Autodesk Inventor part; units mm, degrees
ref_plane "YZ Plane" through (0, 0, 0) normal (1, 0, 0) x (0, 1, 0)
ref_plane "XZ Plane" through (0, 0, 0) normal (0, 1, 0) x (-1, 0, 0)
ref_plane "XY Plane" through (0, 0, 0) normal (0, 0, 1) x (1, 0, 0)
sketch "Sketch1" plane through (0, 0, 0) normal (0, 1, 0) x (-1, 0, 0)
  arc A0 (32.2948, 13.759) -> (-8.6569, 13.759) centre (11.8189, 4.9346) ccw
  line L0 (-8.6569, 13.759) -> (-8.6569, -3.8898)
  line L1 (-1.7811, -3.8898) -> (-8.6569, -3.8898)
  line L2 (-1.7811, -3.8898) -> (-1.7811, -10.2398)
  line L3 (-1.7811, -10.2398) -> (4.2189, -10.2398)
  line L4 (4.2189, -10.2398) -> (4.2189, -3.8898)
  line L5 (10.3189, -3.8898) -> (4.2189, -3.8898)
  line L6 (10.3189, -3.8898) -> (10.3189, 2.1102)
  line L7 (10.3189, 2.1102) -> (9.0689, 2.1102)
  line L8 (9.0689, 2.1102) -> (9.0689, 4.1102)
  line L9 (9.0689, 4.1102) -> (10.3189, 4.1102)
  line L10 (10.3189, 4.1102) -> (10.3189, 6.7602)
  line L11 (10.3189, 6.7602) -> (13.3189, 6.7602)
  line L12 (13.3189, 6.7602) -> (13.3189, 4.1102)
  line L13 (13.3189, 4.1102) -> (14.5689, 4.1102)
  line L14 (14.5689, 4.1102) -> (14.5689, 2.1102)
  line L15 (14.5689, 2.1102) -> (13.3189, 2.1102)
  line L16 (13.3189, 2.1102) -> (13.3189, -3.8898)
  line L17 (19.4189, -3.8898) -> (13.3189, -3.8898)
  line L18 (19.4189, -3.8898) -> (19.4189, -10.2398)
  line L19 (19.4189, -10.2398) -> (25.4189, -10.2398)
  line L20 (25.4189, -10.2398) -> (25.4189, -3.8898)
  line L21 (32.2948, -3.8898) -> (25.4189, -3.8898)
  line L22 (32.2948, -3.8898) -> (32.2948, 13.759)
  circle A1 centre (11.8189, 11.3099) radius 4
  line L23 (-7.9734, -40.7116) -> (-7.9734, -55.3652)
  line L24 (-1.0976, -55.3652) -> (-7.9734, -55.3652)
  line L25 (-1.0976, -55.3652) -> (-1.0976, -61.7152)
  line L26 (-1.0976, -61.7152) -> (4.9025, -61.7152)
  line L27 (4.9025, -61.7152) -> (4.9025, -55.3652)
  line L28 (11.0025, -55.3652) -> (4.9025, -55.3652)
  line L29 (11.0025, -55.3652) -> (11.0025, -49.3652)
  line L30 (11.0025, -49.3652) -> (9.7525, -49.3652)
  line L31 (9.7525, -49.3652) -> (9.7525, -47.3652)
  line L32 (9.7525, -47.3652) -> (11.0025, -47.3652)
  line L33 (11.0025, -47.3652) -> (11.0025, -44.7152)
  line L34 (11.0025, -44.7152) -> (14.0025, -44.7152)
  line L35 (14.0025, -44.7152) -> (14.0025, -47.3652)
  line L36 (14.0025, -47.3652) -> (15.2524, -47.3652)
  line L37 (15.2524, -47.3652) -> (15.2524, -49.3652)
  line L38 (15.2524, -49.3652) -> (14.0025, -49.3652)
  line L39 (14.0025, -49.3652) -> (14.0025, -55.3652)
  line L40 (20.1024, -55.3652) -> (14.0025, -55.3652)
  line L41 (20.1024, -55.3652) -> (20.1024, -61.7152)
  line L42 (20.1024, -61.7152) -> (26.1024, -61.7152)
  line L43 (26.1024, -61.7152) -> (26.1024, -55.3652)
  line L44 (32.9783, -55.3652) -> (26.1024, -55.3652)
  line L45 (32.9783, -55.3652) -> (32.9783, -40.7116)
  line L46 (32.9783, -40.7116) -> (-7.9734, -40.7116)
  point P0 (0, 0)
  point P1 (0.6835, -51.4754)
  point P2 (12.5025, -46.5408)
extrude "Extrusion1" add sketch "Sketch1" along normal blind 6 contours L46 L45 L44 L43 L42 L41 L40 L39 L38 L37 L36 L35 L34 L33 L32 L31 L30 L29 L28 L27 L26 L25 L24 L23
sketch "Sketch2" plane through (0, 6, 0) normal (0, 1, 0) x (1, 0, 0)
  line L0 (-14.0025, 49.3652) -> (-14.0025, 55.3652)
  line L1 (-15.2524, 47.3652) -> (-15.2524, 49.3652)
  line L2 (-15.2524, 49.3652) -> (-14.0025, 49.3652)
  line L3 (-14.0025, 47.3652) -> (-15.2524, 47.3652)
  line L4 (-14.0025, 44.7152) -> (-14.0025, 47.3652)
  line L5 (-11.0025, 44.7152) -> (-14.0025, 44.7152)
  line L6 (-11.0025, 47.3652) -> (-11.0025, 44.7152)
  line L7 (-9.7525, 47.3652) -> (-11.0025, 47.3652)
  line L8 (-9.7525, 49.3652) -> (-9.7525, 47.3652)
  line L9 (-11.0025, 49.3652) -> (-9.7525, 49.3652)
  line L10 (-11.0025, 55.3652) -> (-11.0025, 49.3652)
  line L11 (-4.9025, 55.3652) -> (-11.0025, 55.3652)
  line L12 (-11.0025, 55.3652) -> (-14.0025, 55.3652)
  line L13 (-14.2025, 47.1652) -> (-15.4524, 47.1652)
  line L14 (-15.4524, 47.1652) -> (-15.4524, 49.5652)
  line L15 (-15.4524, 49.5652) -> (-14.2025, 49.5652)
  line L16 (-14.2025, 49.5652) -> (-14.2025, 55.5652)
  line L17 (-14.2025, 55.5652) -> (-10.8025, 55.5652)
  line L18 (-10.8025, 55.5652) -> (-10.8025, 49.5652)
  line L19 (-10.8025, 49.5652) -> (-9.5525, 49.5652)
  line L20 (-9.5525, 49.5652) -> (-9.5525, 47.1652)
  line L21 (-9.5525, 47.1652) -> (-10.8025, 47.1652)
  line L22 (-10.8025, 47.1652) -> (-10.8025, 44.5152)
  line L23 (-10.8025, 44.5152) -> (-14.2025, 44.5152)
  line L24 (-14.2025, 44.5152) -> (-14.2025, 47.1652)
  point P0 (0, 0)
  dimension "d2" = 0.2
extrude "Extrusion2" cut sketch "Sketch2" against normal blind 25.4
sketch "Sketch3" plane through (0, 6, 0) normal (0, 1, 0) x (1, 0, 0)
  line L0 (2.9926, 65.1915) -> (-28.8734, 65.1915)
  line L1 (-28.8734, 65.1915) -> (-28.8734, 59.7152)
  line L2 (-28.8734, 59.7152) -> (2.9926, 59.7152)
  line L3 (2.9926, 59.7152) -> (2.9926, 65.1915)
  line L4 (-20.1024, 61.7152) -> (-26.1024, 61.7152)
  point P0 (0, 0)
  dimension "d5" = 2
extrude "Extrusion3" cut sketch "Sketch3" against normal blind 25.4
fillet "Fillet1" radius 0.5 4 edges at (-26.1024, 3, -59.7152) (-20.1024, 3, -59.7152) (-4.9025, 3, -59.7152) (1.0976, 3, -59.7152)
properties part number "Maker_jigsaw_template"
Can you work these out from the model? Positions are in its coordinate system, mm. A direction names the side the tool comes from. Round coordinates to 2 decimals unless told otherwise and drop trailing zeros. Loops run counter-clockwise (first coordinate to the right, second up) from the corner with the lowest first, then second, coordinate; pieces in that order, holes last. Notation, with made-up numbers: M 14,89.25 L 50,89.25 A29 cw 50,112.25 Z; hole C 23,-2 d11. An arc over 180 degrees is marked long. Answer as a JSON object with one key per item and string values. Group by question number.
Q1. Imagine slicing it at C-C, the plane z = -50. Please give me the cut outline in (x, y).
Q2. We'd pull the mould along X, two halves only. Please class faces 1 (the flat face through (-13, 3, -40.712)), 2 (the flat face through (-26.102, 3, -57)), 3 (the flat face through (1.098, 3, -57)), 4 (the flat face through (-10, 3, -49.565)): +X half, -X half, draft (parallel to the pull), parting line (faces both ways), or undercut.
Q3. On a 3-axis mill with a long thin cutter (end or side, diameter ignored), from which of +Z, -Z, +X, -X, +Y, -Y can I reach the whole of each face in a straight line? I mean faces 5 (the flat face through (4, 3, -55.365)), 6 (the flat face through (-15, 3, -47.165)), 7 (the flat face through (-8, 3, -55.365)). Say none if no direction works.
Q4. Please list where these lines run through material, in increasing order: L1, parallel to X at y = 2.1, z = -46; L2, parallel to X at y = 1.5, z = -55.5; L3, parallel to Z at x = -14, y = 1.1.
Q5. Will these pins go through, and if not, where does the flat tip stop? pin 1 (1.4 mm diameter, centred on x = -14.5, y = 3, fed in from -Z); pin 2 (1.2 mm diameter, centred on y = 2, z = -57, fed in from +X).
Q6. Imagine slicing it at A-A, the plane z = -58.25. Please give me the cut outline in (x, y).
Q7. Imagine slicing it at B-B, the plane y = 1.1. Please give me the cut outline in (x, z).
Q8. Imagine slicing it at D-D, the plane x = -16.5. Please give me the cut outline in (y, z), then the cut area to 3 significant figures.
Findings:
{
 "1": {"outline": "M -32.98,0 L -14.2,0 L -14.2,6 L -32.98,6 Z; M -10.8,0 L 7.97,0 L 7.97,6 L -10.8,6 Z"},
 "2": {"face 1": "draft", "face 2": "-X half", "face 3": "+X half", "face 4": "undercut"},
 "3": {"face 5": "-Z, +X, +Y, -Y", "face 6": "+Y, -Y", "face 7": "-Z, +Y, -Y"},
 "4": {"L1": "x = -32.98 to -14.2, -10.8 to 7.97", "L2": "x = -26.1 to -20.1, -4.9 to 1.1", "L3": "z = -44.52 to -40.71"},
 "5": {"pin 1": "stops at z = -55.37", "pin 2": "stops at x = 1.1"},
 "6": {"outline": "M -26.1,0 L -20.1,0 L -20.1,6 L -26.1,6 Z; M -4.9,0 L 1.1,0 L 1.1,6 L -4.9,6 Z"},
 "7": {"outline": "M -32.98,-55.37 L -26.1,-55.37 L -26.1,-59.22 A0.5 ccw -25.6,-59.72 L -20.6,-59.72 A0.5 ccw -20.1,-59.22 L -20.1,-55.37 L -14.2,-55.37 L -14.2,-49.57 L -15.45,-49.57 L -15.45,-47.17 L -14.2,-47.17 L -14.2,-44.52 L -10.8,-44.52 L -10.8,-47.17 L -9.55,-47.17 L -9.55,-49.57 L -10.8,-49.57 L -10.8,-55.37 L -4.9,-55.37 L -4.9,-59.22 A0.5 ccw -4.4,-59.72 L 0.6,-59.72 A0.5 ccw 1.1,-59.22 L 1.1,-55.37 L 7.97,-55.37 L 7.97,-40.71 L -32.98,-40.71 Z"},
 "8": {"outline": "M 0,-55.37 L 6,-55.37 L 6,-40.71 L 0,-40.71 Z", "area": "87.9 mm2"}
}
